Verification items for the finished model (mm, model axes). Give positions to 0.01 mm unless a question says otherwise; leave off trailing zeros. Loops run counter-clockwise (first coordinate to the right, second up) from the corner with the lowest first, then second, coordinate; pieces in that order, holes last. Notation, with made-up numbers: (2, -24) - (58, -24) arc R16 cw to (58, -15) - close; hole circle Ø7 at (23, 40). An arc over 180 degrees is marked (long way). Answer in a Markdown table with one row per item.
```python
from build123d import *

# Parameters (mm, degrees)
BASE_FLANGE1_DEPTH = 6.35
SKETCH8_R          = 3.4
CUT_EXTRUDE1_DEPTH = 175.95180765


# Sheet-metal steps are written as plain solids
with BuildPart() as part:
    # Sketch2 → Base-Flange1 (new body)
    with BuildSketch(Plane(origin=(0, 0, 0), x_dir=(1, 0, 0), z_dir=(0, 1, 0))):
        with BuildLine():
            Line((0, 0), (38.51093065, 0))
            Line((38.51093065, 0), (95.630465325, 57.119534675))
            ThreePointArc((95.630465325, 57.119534675), (99.287953618, 118.761570635), (38.51093065, 129.682710556))
            Line((38.51093065, 129.682710556), (0, 90))
            Line((0, 90), (0, 0))
        make_face()
    extrude(amount=-BASE_FLANGE1_DEPTH)

    # Sketch8 → Cut-Extrude1 (cut, through all)
    with BuildSketch(Plane(origin=(0, 0, 0), x_dir=(1, 0, 0), z_dir=(0, 1, 0))):
        with Locations(Location((12.5, 79, 0), (0, 0, 270))):
            Circle(SKETCH8_R)
        with Locations(Location((12.5, 11, 0), (0, 0, 90))):
            Circle(SKETCH8_R)
    extrude(amount=-CUT_EXTRUDE1_DEPTH, mode=Mode.SUBTRACT)


solid = part.part
```
Q1. Sectioned sample at A-A (y = -3.75). Record the cut outline in (x, z), and give its area (3 significant figures).
Completed:
| item | result |
|---|---|
| outline | (0, -90) - (38.51, -129.68) arc R46.5 ccw to (95.63, -57.12) - (38.51, 0) - (0, 0) - close; hole circle Ø6.8 at (12.5, -79); hole circle Ø6.8 at (12.5, -11) |
| area | 10,700 mm^2 |
Q2. Thickness scan on line 1 (X direction, y = -3.25, z = -11); line 2 (X direction, y = -2.75, z = -79); line 3 (Z direction, x = 38.5, y = -1.25). Record the ranges inside material, lowest first.
Completed:
| item | result |
|---|---|
| line 1 | 0 to 9.1, 15.9 to 49.51 |
| line 2 | 0 to 9.1, 15.9 to 107.93 |
| line 3 | -129.67 to 0 |
Q3. Sectioned sample at D-D (z = -79). Record the cut outline in (x, y).
Completed:
| item | result |
|---|---|
| outline | (0, -6.35) - (9.1, -6.35) - (9.1, 0) - (0, 0) - close; (15.9, -6.35) - (107.93, -6.35) - (107.93, 0) - (15.9, 0) - close |
Q4. Draft check along Z on faces 1 (the face through (10.431, -3.131, -81.698)), 2 (the face through (0, -3, -46)), 3 (the face through (19, -3, 0)). Enter one of: +Z half, -Z half, draft (parallel to the pull), parting line (faces both ways), or undercut.
Completed:
| item | result |
|---|---|
| face 1 | undercut |
| face 2 | draft |
| face 3 | +Z half |
Q5. Go/stop test with a flat-tipped pin: P1, Ø2, axis at x = 40, y = -5, coming from the -Z side. Record where the tip stops, or that it passes through.
Completed:
| item | result |
|---|---|
| P1 | z = -131.1 |
Q6. Sectioned sample at C-C (x = 12.5). Record the cut outline in (y, z), and give its area (3 significant figures).
Completed:
| item | result |
|---|---|
| outline | (-6.35, -102.88) - (0, -102.88) - (0, -82.4) - (-6.35, -82.4) - close; (-6.35, -75.6) - (0, -75.6) - (0, -14.4) - (-6.35, -14.4) - close; (-6.35, -7.6) - (0, -7.6) - (0, 0) - (-6.35, 0) - close |
| area | 567 mm^2 |
Q7. Sectioned sample at B-B (z = -11). Record the cut outline in (x, y), and give its area (3 significant figures).
Completed:
| item | result |
|---|---|
| outline | (0, -6.35) - (9.1, -6.35) - (9.1, 0) - (0, 0) - close; (15.9, -6.35) - (49.51, -6.35) - (49.51, 0) - (15.9, 0) - close |
| area | 271 mm^2 |
